Read the model definition and answer for the solid it produces. Units are mm, in the model's axes. Face numbers are marked on the shaded views. Coordinates: 2 decimals unless noted, no trailing zeros. Write each loop counter-clockwise with the first axis right and the second up, starting at its lowest first coordinate (ties: lowest second). Pieces come first, ordered by that corner, then holes. Notation, with made-up numbers: (-37.5, 67) - (-33.5, 67) arc R17 cw to (-33.5, 81) - close; hole circle Ø9 at (38.5, 82.25). An arc over 180 degrees is marked (long way). Use a Markdown table: item, result.
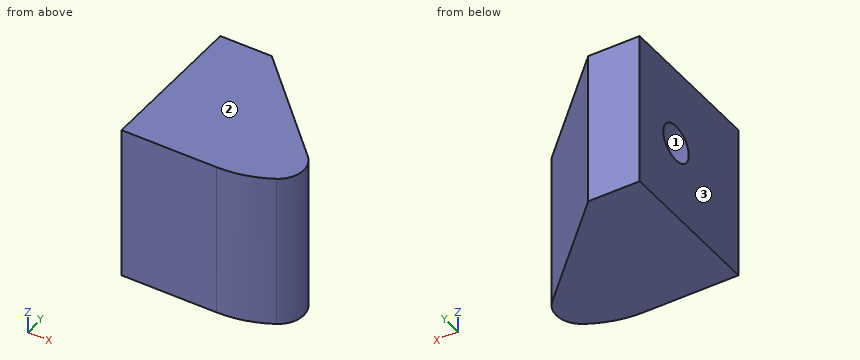
from build123d import *

# Parameters (mm, degrees)
F1_DEPTH    = 300
F2_T1_DEPTH = 778.5765609082
F3_R        = 50
F5_R        = 35
F6_DEPTH    = 250


# Not quite as in the source:
# - a fillet or chamfer that OpenCascade refuses, or shapes differently, is made with other operations: its cross-section is extruded or revolved along the edge and cut away or added


with BuildPart() as f1:
    # F0 (on Top) → F1 (new body)
    with BuildSketch(Plane.XY):
        Polygon((0, 300), (0, 0), (280, 0), (333.3452377916, 66.6547622084), (100, 300), align=None)
    extrude(amount=-F1_DEPTH)

    # F2: fillet of radius 200 on 1 edges, made by hand

    # F2_s2 → F2_t1 (cut)
    with BuildSketch(Plane.XY.offset(-539.2882804541)):
        with BuildLine():
            ThreePointArc((184.2846878184, 0), (265.9270556236, 17.4225540239), (333.3452377916, 66.6547622084))
            Line((333.3452377916, 66.6547622084), (280, 0))
            Line((280, 0), (184.2846878184, 0))
        make_face()
    extrude(amount=F2_T1_DEPTH, mode=Mode.SUBTRACT)

    # F3
    f3_edges = [f1.edges().sort_by_distance(p)[0] for p in [
        (333.345238, 66.654762, -150),
    ]]
    fillet(f3_edges, radius=F3_R)

    # F5 (on face) → F6 (cut)
    with BuildSketch(Plane(origin=(-114.9066664678, 53.581858547, 0), x_dir=(-0.4226182617, -0.906307787, 0), z_dir=(-0.906307787, 0.4226182617, 0))):
        with Locations((-171.892336111, -150)):
            Circle(F5_R)
    extrude(amount=-F6_DEPTH, mode=Mode.SUBTRACT)


solid = f1.part
(1) A cutting plane is placed at B-B, the plane z = -212. Write down the section's boundary in (x, y).
Report:
| item | result |
|---|---|
| outline | (0, 0) - (184.28, 0) arc R200 ccw to (284.21, 26.75) arc R50 ccw to (294.58, 105.42) - (100, 300) - (0, 300) - close |
(2) Each of these flat-tipped pins is pushed along its axis until it touches: P1, Ø6, axis at y = 149, z = -77.5, coming from the +X side; P2, Ø2, axis at x = 185.5, z = -152, coming from the -Y side; P3, Ø1, axis at x = 207.5, z = -117.5, coming from the -Y side; P4, Ø3, axis at x = 176, y = 142, coming from the +Z side. Where does it stop, or does it pass through?
Report:
| item | result |
|---|---|
| P1 | stops at x = 254 |
| P2 | stops at y = 0 |
| P3 | stops at y = 1.29 |
| P4 | stops at z = 0 |
(3) A cutting plane is placed at A-A, the plane y = 250. Write down the section's boundary in (x, z), and give its area (3 significant figures).
Report:
| item | result |
|---|---|
| outline | (0, -300) - (150, -300) - (150, 0) - (0, 0) - close |
| area | 45,000 mm² |
(4) A cutting plane is placed at C-C, the plane x = 213. Write down the section's boundary in (y, z), and give its area (3 significant figures).
Report:
| item | result |
|---|---|
| outline | (2.07, -300) - (187, -300) - (187, 0) - (2.07, 0) - close |
| area | 55,500 mm² |
(5) A cutting plane is placed at D-D, the plane z = -162. Write down the section's boundary in (x, y), and give its area (3 significant figures).
Report:
| item | result |
|---|---|
| outline | (0, 0) - (184.28, 0) arc R200 ccw to (284.21, 26.75) arc R50 ccw to (294.58, 105.42) - (100, 300) - (0, 300) - (0, 225.94) - (198.21, 133.51) - (170.42, 73.92) - (0, 153.38) - close |
| area | 55,600 mm² |
(6) The mould has two halves that part along X. Classify the marked faces 1, 2 and 3: pulls with the +X half, pulls with the -X half, needs draft (parallel to the pull), parting line crosses it, or undercut.
Report:
| item | result |
|---|---|
| face 1 | undercut |
| face 2 | needs draft |
| face 3 | pulls with the -X half |
(7) Straight lines are drawn through the part: L1, parallel to Y at x = 169, z = -150.5; L2, parallel to Z at x = 63, y = 140.5; L3, parallel to X at y = 91, z = -132.5. For each, find the intervals that lie inside material, in ascending order.
Report:
| item | result |
|---|---|
| L1 | y = 0 to 72.24, 149.47 to 231 |
| L2 | z = -300 to -180.06, -119.94 to 0 |
| L3 | x = 0 to 139.86, 178.39 to 304.63 |
